Design review of the part built by this model. Coordinates are the model's own, in mm. A direction names the side the tool comes from. Give positions to 0.01 mm unless a question says otherwise; leave off trailing zeros. Order: outer loops, then holes, each group sorted by start corner. A loop starts at its lowest first (then second) coordinate and runs counter-clockwise, first axis right, second up. Notation, with made-up numbers: (7, -2) -> (57, -2) arc R28 cw to (57, 35) -> close; hole circle Ø2 at (-15, 46). An arc over 180 degrees is marked (long way). One line per item, written item: value.
from build123d import *

# Parameters (mm, degrees)
F1_DEPTH = 50.8
F3_D     = 63.5


with BuildPart() as f1:
    # F0 (on Front) → F1 (new body)
    with BuildSketch(Plane.XZ):
        with BuildLine():
            ThreePointArc((-25.4, -30.7949761419), (-15.5542598667, -93.9734218577), (38.1, -59.1930394562))
            ThreePointArc((38.1, -59.1930394562), (34.7803824016, -43.6387795895), (25.4, -30.7949761419))
            Line((25.4, -30.7949761419), (25.4, -47.553297191))
            Line((25.4, -47.553297191), (-25.4, -47.553297191))
            Line((-25.4, -47.553297191), (-25.4, -30.7949761419))
        make_face()
        with BuildLine():
            Line((25.4, -47.553297191), (25.4, -30.7949761419))
            ThreePointArc((25.4, -30.7949761419), (0, -21.0930394562), (-25.4, -30.7949761419))
            Line((-25.4, -30.7949761419), (-25.4, -47.553297191))
            Line((-25.4, -47.553297191), (25.4, -47.553297191))
        make_face()
        with BuildLine():
            ThreePointArc((-25.4, -30.7949761419), (0, -21.0930394562), (25.4, -30.7949761419))
            Line((25.4, -30.7949761419), (25.4, 28.646702809))
            Line((25.4, 28.646702809), (-25.4, 28.646702809))
            Line((-25.4, 28.646702809), (-25.4, -30.7949761419))
        make_face()
    extrude(amount=F1_DEPTH)

    # F3 (through all)
    with Locations(Plane.XZ.offset(50.8)):
        with Locations((0, -59.1930394562)):
            Hole(F3_D / 2)


solid = f1.part
Item 1: Add section D-D on z = 11. Give the boundary of the cut face in (x, y), plus the area to 3 significant figures.
Returned:
outline: (-25.4, -50.8) -> (25.4, -50.8) -> (25.4, 0) -> (-25.4, 0) -> close
area: 2,580 mm²
Item 2: Add section A-A on x = 0. Give the boundary of the cut face in (y, z).
Returned:
outline: (-50.8, -97.29) -> (0, -97.29) -> (0, -90.94) -> (-50.8, -90.94) -> close; (-50.8, -27.44) -> (0, -27.44) -> (0, 28.65) -> (-50.8, 28.65) -> close
Item 3: Add section C-C on y = -26. Give the boundary of the cut face in (x, z).
Returned:
outline: (-25.4, -30.79) arc R38.1 ccw (long way) to (25.4, -30.79) -> (25.4, 28.65) -> (-25.4, 28.65) -> close; hole circle Ø63.5 at (0, -59.19)
Item 4: Draft analysis for pull direction Z (two halves, no side actions). For faces 4 (the cylindrical face through (-1.29, -25.04, -97.27)), 5 (the flat face through (0, -25, 28.647)), 6 (the cylindrical face through (-30.284, -25.044, -49.656)), 7 (the flat face through (-1, 0, -19)), state which applies: pulls with the +Z half, pulls with the -Z half, needs draft (parallel to the pull), parting line crosses it, or undercut.
Returned:
face 4: parting line crosses it
face 5: pulls with the +Z half
face 6: undercut
face 7: needs draft
Item 5: Machinability: for faces 1 (the flat face through (-25.4, -25, -1)), 2 (the flat face through (25.4, -25, -1)), 3 (the flat face through (-1, -50.8, -19)), which of the approach directions +Z, -Z, +X, -X, +Y, -Y give a long, thin tool a straight path to every point of the face, cutting with its end or side? Answer none if there is none.
Returned:
face 1: +Z, -X, +Y, -Y
face 2: +Z, +X, +Y, -Y
face 3: +Z, -Z, +X, -X, -Y
Item 6: To check wall thickness, follow line 1 along Z through (x, y) = (0, -27); line 2 along X through (y, z) = (-14.5, 1.5); line 3 along Z through (x, y) = (29, -16). State the ranges of each line that lie inside material, in increasing order. Write a range as from..to.
Returned:
line 1: -97.29..-90.94, -27.44..28.65
line 2: -25.4..25.4
line 3: -83.9..-72.12, -46.27..-34.48
Item 7: Add section B-B on z = -51.5. Give the boundary of the cut face in (x, y), plus the area to 3 significant figures.
Returned:
outline: (-37.32, -50.8) -> (-30.8, -50.8) -> (-30.8, 0) -> (-37.32, 0) -> close; (30.8, -50.8) -> (37.32, -50.8) -> (37.32, 0) -> (30.8, 0) -> close
area: 662 mm²
Item 8: Clearance check with flat-ended pins moving along their axes: P1, Ø2, axis at y = -25, z = -12.5, coming from the -X side; P2, Ø5, axis at y = -7.5, z = -32.5, coming from the -X side; P3, Ø5, axis at y = -9, z = -38.5, coming from the -X side. State where each tip first meets the part, or that it passes through.
Returned:
P1: x = -25.4
P2: x = -29.43
P3: x = -33.48
